```python
from build123d import *

# Parameters (mm, degrees)
F1_DEPTH = 7
F3_DEPTH = 34.2
F4_R     = 1.75
F5_DEPTH = 4
F6_R     = 4
F7_DEPTH = 25
F8_R     = 3
F9_DEPTH = 1.1867513459


with BuildPart() as f1:
    # F0 (on Front) → F1 (new body)
    with BuildSketch(Plane.XZ):
        Polygon((14, 2.8867513459), (5, 2.8867513459), (5, -2.8867513459), (0, -5.7735026919), (-5, -2.8867513459), (-5, 2.8867513459), (-14, 2.8867513459), (-14, -9.6132486541), (14, -9.6132486541), align=None)
    extrude(amount=F1_DEPTH)

    # F2 (on face) → F3 (cut)
    with BuildSketch(Plane.YZ.offset(14)):
        with BuildLine():
            ThreePointArc((-4.425, 0), (-3, -1.425), (-1.575, 0))
            Line((-1.575, 0), (-4.425, 0))
        make_face()
        with BuildLine():
            Line((-4.425, 0), (-1.575, 0))
            ThreePointArc((-1.575, 0), (-3, 1.425), (-4.425, 0))
        make_face()
    extrude(amount=-F3_DEPTH, mode=Mode.SUBTRACT)

    # F4 (on face) → F5 (join)
    with BuildSketch(Plane(origin=(0, 0, 0), x_dir=(-1, 0, 0), z_dir=(0, 1, 0))):
        with BuildLine():
            ThreePointArc((-5.1, -6.8), (-8.1441186755, -2.4337894321), (-7.9947899701, 2.8867513459))
            Line((-7.9947899701, 2.8867513459), (-14, 2.8867513459))
            Line((-14, 2.8867513459), (-19, -6.8))
            ThreePointArc((-19, -6.8), (-17.8284271247, -9.6284271247), (-15, -10.8))
            Line((-15, -10.8), (15, -10.8))
            ThreePointArc((15, -10.8), (17.8284271247, -9.6284271247), (19, -6.8))
            Line((19, -6.8), (14, 2.8867513459))
            Line((14, 2.8867513459), (7.9947899701, 2.8867513459))
            ThreePointArc((7.9947899701, 2.8867513459), (5.0550212811, -6.833502751), (-5.1, -6.8))
        make_face()
        with Locations((-15, -6.8)):
            Circle(F4_R, mode=Mode.SUBTRACT)
        with Locations((15, -6.8)):
            Circle(F4_R, mode=Mode.SUBTRACT)
    extrude(amount=F5_DEPTH)

    # F6 (on face) → F7 (cut)
    with BuildSketch(Plane.XZ):
        with Locations((-15, -6.8)):
            Circle(F6_R)
        with Locations((15, -6.8)):
            Circle(F6_R)
    extrude(amount=F7_DEPTH, mode=Mode.SUBTRACT)

    # F8
    f8_edges = [f1.edges().sort_by_distance(p)[0] for p in [
        (-12.156475, -3.5, -9.613249),
        (12.156475, -3.5, -9.613249),
    ]]
    fillet(f8_edges, radius=F8_R)

    # F9 (add, through all): a face of the model
    f9_faces = [f1.faces().sort_by_distance(p)[0] for p in [
        (0, -3.5, -9.6132486541),
    ]]
    extrude(f9_faces, amount=F9_DEPTH)


solid = f1.part
```
CAD build for the part. Positions are in the model's coordinates, mm. A direction names the side the tool comes from. Round coordinates to 2 decimals unless told otherwise and drop trailing zeros. Write each loop counter-clockwise with the first axis right and the second up, starting at its lowest first coordinate (ties: lowest second). Pieces come first, ordered by that corner, then holes. Notation, with made-up numbers: (18.5, 73.25) - (41.5, 73.25) arc R8 cw to (41.5, 81.25) - close; hole circle Ø6 at (-17.5, 11). An arc over 180 degrees is marked (long way). Write item = value, one per line. Start each with the question number.
Q1. Band-saw the part on A-A (y = -3). Give the cut face in (x, z) (1 decimal), then the cut area to 3 significant figures.
Q2. Which spindle directions (+Z, -Z, +X, -X, +Y, -Y) get a long thin tool onto all of the face, cutting with end or side? Do faces 4 (the flat face through (8.002, -4, -10)), 5 (the flat face through (-14, -5, 0)), 6 (the flat face through (2.535, -3.451, -4.31)), 7 (the flat face through (-13, 0, -6)), 8 (the cylindrical face through (13.383, 1.972, -7.47)). Say none if no direction does.
Q3. Band-saw the part on B-B (z = -8). Give the cut face in (x, y), then the cut area to 3 significant figures.
Q4. Probe L1, parallel to Z at x = 7.5, y = -3 (3 decimals); L2, parallel to X at y = -0.75, z = 1.75; L3, parallel to X at y = 0.85, z = -6.8. List the from-to ranges inside material, lowest first. Write a range as from..to.
Q5. Mould opens along Y. For faces 1 (the cylindrical face through (-9.44, -1.64, 0.43)), 2 (the cylindrical face through (17.859, 1.972, -9.597)), 3 (the flat face through (0, 4, -10)) say: pulls with the +Y half, pulls with the -Y half, needs draft (parallel to the pull), parting line crosses it, or undercut.
Q6. Band-saw the part on D-D (z = 0). Give the cut face in (x, y) (3 decimals).
Q7. Band-saw the part on C-C (x = 7.5). Give the cut face in (y, z) (3 decimals).
Q8. Drop flat-ended pins along their axis: pin 1 (4.5 mm diameter, centred on y = -4.5, z = 0.5, fed in from +X); pin 2 (4.5 mm diameter, centred on y = -3.5, z = 1, fed in from -X); pin 3 (0.6 mm diameter, centred on y = -2.5, z = -10.5, fed in from +X). Give the stop position or say it passes through.
Answers below:
q1.outline = (-14, -2.9) arc R4 cw to (-11, -6.7) arc R3 ccw to (-8, -9.6) - (-8, -10.8) - (8, -10.8) - (8, -9.6) arc R3 ccw to (11, -6.7) arc R4 cw to (14, -2.9) - (14, -1.4) - (5, -1.4) - (5, -2.9) - (0, -5.8) - (-5, -2.9) - (-5, -1.4) - (-14, -1.4) - close; (-14, 1.4) - (-5, 1.4) - (-5, 2.9) - (-14, 2.9) - close; (5, 1.4) - (14, 1.4) - (14, 2.9) - (5, 2.9) - close
q1.area = 208 mm2
q2.face_4 = -Z, +X, -Y
q2.face_5 = +Z, -Z, -X, -Y
q2.face_6 = +Z, +Y, -Y
q2.face_7 = -Z, -X, -Y
q2.face_8 = +Y, -Y
q3.outline = (-18.82, 0) - (-16.27, 0) - (-16.27, 4) - (-18.82, 4) - close; (-13.73, 0) - (-10.66, 0) - (-10.66, -7) - (10.66, -7) - (10.66, 0) - (13.73, 0) - (13.73, 4) - (2.87, 4) - (2.87, 0) - (-2.87, 0) - (-2.87, 4) - (-13.73, 4) - close; (16.27, 0) - (18.82, 0) - (18.82, 4) - (16.27, 4) - close
q3.area = 256 mm2
q4.L1 = -10.8..-1.425, 1.425..2.887
q4.L2 = -14..-5, 5..14
q4.L3 = -19..-16.75, -13.25..-5.1, 5.1..13.25, 16.75..19
q5.face_1 = undercut
q5.face_2 = needs draft
q5.face_3 = pulls with the +Y half
q6.outline = (-15.49, 0) - (-14, 0) - (-14, -1.575) - (-5, -1.575) - (-5, 0) - (-8.5, 0) - (-8.5, 4) - (-15.49, 4) - close; (-14, -7) - (-5, -7) - (-5, -4.425) - (-14, -4.425) - close; (5, -7) - (14, -7) - (14, -4.425) - (5, -4.425) - close; (5, -1.575) - (14, -1.575) - (14, 0) - (15.49, 0) - (15.49, 4) - (8.5, 4) - (8.5, 0) - (5, 0) - close
q7.outline = (-7, -10.8) - (4, -10.8) - (4, -4) - (0, -4) - (0, 2.887) - (-7, 2.887) - close; hole circle Ø2.85 at (-3, 0)
q8.pin_1 = 14
q8.pin_2 = -14
q8.pin_3 = 8
